from build123d import *

# Parameters (mm, degrees)
SALIENTE_EXTRUIR1_DEPTH  = 38
CORTAR_EXTRUIR1_DEPTH    = 273.053680503
CROQUIS3_R               = 19
SALIENTE_EXTRUIR3_DEPTH  = 26
REDONDEO1_R              = 6
CROQUIS4_R               = 28.5
CORTAR_EXTRUIR2_DEPTH    = 1
REDONDEO1_OF_SIMETR_A1_R = 6
REDONDEO2_R              = 6


with BuildPart() as part:
    # Croquis1 → Saliente-Extruir1 (new, symmetric)
    with BuildSketch(Plane.XY):
        Polygon((0, 0), (0, 139), (38, 139), (127, 50), (127, 0), align=None)
    extrude(amount=SALIENTE_EXTRUIR1_DEPTH, both=True)

    # Croquis2 → Cortar-Extruir1 (cut, through all, along a direction that is not the sketch's normal)
    with BuildSketch(Plane(origin=(0, 139, 0), x_dir=(1, 0, 0), z_dir=(0, 1, 0))):
        Polygon((38, 0), (38, 13), (12, 13), (12, -13), (38, -13), align=None)
    extrude(amount=-CORTAR_EXTRUIR1_DEPTH, dir=(-0.7071067811865515, 0.7071067811865436, 0), mode=Mode.SUBTRACT)

    # Croquis3 → Saliente-Extruir3 (add)
    with BuildSketch(Plane.XZ):
        with BuildLine():
            Line((0, 38), (0, 89))
            ThreePointArc((0, 89), (38, 127), (76, 89))
            Line((76, 89), (76, 38))
            Line((76, 38), (0, 38))
        make_face()
        with Locations((38, 89)):
            Circle(CROQUIS3_R, mode=Mode.SUBTRACT)
    saliente_extruir3 = extrude(amount=-SALIENTE_EXTRUIR3_DEPTH)

    # Redondeo1
    redondeo1_edges = [part.edges().sort_by_distance(p)[0] for p in [
        (38, 26, 127),
        (76, 26, 63.5),
        (0, 26, 63.5),
    ]]
    fillet(redondeo1_edges, radius=REDONDEO1_R)

    # Croquis4 → Cortar-Extruir2 (cut)
    with BuildSketch(Plane(origin=(0, 26, 0), x_dir=(1, 0, 0), z_dir=(0, 1, 0))):
        with Locations(Location((38, -89, 0), (0, 0, 180))):
            Circle(CROQUIS4_R)
    cortar_extruir2 = extrude(amount=-CORTAR_EXTRUIR2_DEPTH, mode=Mode.SUBTRACT)

    # Simetría1: Saliente-Extruir3, Cortar-Extruir2 across plane
    add(saliente_extruir3.mirror(Plane.XY))
    add(cortar_extruir2.mirror(Plane.XY), mode=Mode.SUBTRACT)

    # Redondeo1 of Simetría1
    redondeo1_of_simetr_a1_edges = [part.edges().sort_by_distance(p)[0] for p in [
        (38, 26, -127),
        (76, 26, -63.5),
        (0, 26, -63.5),
    ]]
    fillet(redondeo1_of_simetr_a1_edges, radius=REDONDEO1_OF_SIMETR_A1_R)

    # Redondeo2
    # the kernel refuses this fillet: 6 mm, written as the material it adds along each edge
    with BuildSketch(Plane(origin=(70, 26, 38), x_dir=(0, 0, 1), z_dir=(-1, 0, 0))) as redondeo2_piece_1:
        with BuildLine():
            CenterArc((REDONDEO2_R, REDONDEO2_R), REDONDEO2_R, 180, 90)
            Line((0, REDONDEO2_R), (0, 0))
            Line((0, 0), (REDONDEO2_R, 0))
        make_face()
    extrude(amount=64)
    with BuildSketch(Plane(origin=(76, 0, 38), x_dir=(0, 0, 1), z_dir=(0, 1, 0))) as redondeo2_piece_2:
        with BuildLine():
            CenterArc((REDONDEO2_R, REDONDEO2_R), REDONDEO2_R, 180, 90)
            Line((0, REDONDEO2_R), (0, 0))
            Line((0, 0), (REDONDEO2_R, 0))
        make_face()
    extrude(amount=20)
    with BuildSketch(Plane(origin=(6, 20, 38), x_dir=(0.8017442392976484, -0.5976672776328276, 0), z_dir=(0.5976672776328276, 0.8017442392976484, 0))) as redondeo2_piece_3_section:
        with BuildLine():
            CenterArc((6 + REDONDEO2_R, -REDONDEO2_R), REDONDEO2_R, 90, 90)
            Line((6 + REDONDEO2_R, 0), (6, 0))
            Line((6, 0), (6, -REDONDEO2_R))
        make_face()
    redondeo2_piece_3 = revolve(axis=Axis((6, 20, 38), (0, 0, -1)), revolution_arc=233.296989237, mode=Mode.PRIVATE)
    redondeo2_piece_3 = split(redondeo2_piece_3, bisect_by=Plane(origin=(0, 24.499633638, 39.86976996), z_dir=(1, 0, 0)), keep=Keep.TOP, mode=Mode.PRIVATE)
    add(redondeo2_piece_3)
    with BuildSketch(Plane(origin=(70, 20, 38), x_dir=(1, 0, 0), z_dir=(0, -1, 0))) as redondeo2_piece_4:
        with BuildLine():
            CenterArc((6 + REDONDEO2_R, REDONDEO2_R), REDONDEO2_R, 180, 90)
            Line((6 + REDONDEO2_R, 0), (6, 0))
            Line((6, 0), (6, REDONDEO2_R))
        make_face()
    revolve(axis=Axis((70, 20, 38), (0, 0, 1)), revolution_arc=90)
    with BuildSketch(Plane(origin=(70, 26, -38), x_dir=(0, 0, -1), z_dir=(-1, 0, 0))) as redondeo2_piece_5:
        with BuildLine():
            CenterArc((REDONDEO2_R, -REDONDEO2_R), REDONDEO2_R, 90, 90)
            Line((0, -REDONDEO2_R), (0, 0))
            Line((0, 0), (REDONDEO2_R, 0))
        make_face()
    extrude(amount=64)
    with BuildSketch(Plane(origin=(76, 0, -38), x_dir=(0, 0, -1), z_dir=(0, 1, 0))) as redondeo2_piece_6:
        with BuildLine():
            CenterArc((REDONDEO2_R, -REDONDEO2_R), REDONDEO2_R, 90, 90)
            Line((0, -REDONDEO2_R), (0, 0))
            Line((0, 0), (REDONDEO2_R, 0))
        make_face()
    extrude(amount=20)
    with BuildSketch(Plane(origin=(6, 20, -38), x_dir=(0.8017442392976486, -0.5976672776328271, 0), z_dir=(0.5976672776328271, 0.8017442392976486, 0))) as redondeo2_piece_7_section:
        with BuildLine():
            CenterArc((6 + REDONDEO2_R, REDONDEO2_R), REDONDEO2_R, 180, 90)
            Line((6, REDONDEO2_R), (6, 0))
            Line((6, 0), (6 + REDONDEO2_R, 0))
        make_face()
    redondeo2_piece_7 = revolve(axis=Axis((6, 20, -38), (0, 0, -1)), revolution_arc=233.296989237, mode=Mode.PRIVATE)
    redondeo2_piece_7 = split(redondeo2_piece_7, bisect_by=Plane(origin=(0, 24.499633653, -39.869769899), z_dir=(1, 0, 0)), keep=Keep.TOP, mode=Mode.PRIVATE)
    add(redondeo2_piece_7)
    with BuildSketch(Plane(origin=(70, 20, -38), x_dir=(1, 0, 0), z_dir=(0, -1, 0))) as redondeo2_piece_8:
        with BuildLine():
            CenterArc((6 + REDONDEO2_R, -REDONDEO2_R), REDONDEO2_R, 90, 90)
            Line((6 + REDONDEO2_R, 0), (6, 0))
            Line((6, 0), (6, -REDONDEO2_R))
        make_face()
    revolve(axis=Axis((70, 20, -38), (0, 0, 1)), revolution_arc=90)


solid = part.part
CAD build for the part. Positions are in the model's coordinates, mm. A direction names the side the tool comes from. Round coordinates to 2 decimals unless told otherwise and drop trailing zeros. Loops run counter-clockwise (first coordinate to the right, second up) from the corner with the lowest first, then second, coordinate; pieces in that order, holes last.
(1) Drop flat-ended pins along their axis: pin 1 (6 mm diameter, centred on x = 104.5, y = 18, fed in from +Z); pin 2 (10 mm diameter, centred on x = 49.5, y = 59.5, fed in from -Z); pin 3 (10 mm diameter, centred on y = 6.5, z = -77.5, fed in from +X). Give the stop position or say it passes through.
(2) Which spindle directions (+Z, -Z, +X, -X, +Y, -Y) get a long thin tool onto all of the face, cutting with end or side? Do faces 1 (the flat face through (76, 10, -67)), 2 (the flat face through (19, 25, 83)), 3 (the cylindrical face through (1.804, 24.289, 66.815)). Say none if no direction does.
(3) Cut at A-A (y = 66.5). Give the cut face in (x, z), plus the area to 3 significant figures.
(4) Cut at B-B (z = 5.5). Give the cut face in (x, y), plus the area to 3 significant figures.
(5) Cut at D-D (x = 41). State how many separate pieces and enclosed holes the cut face has, plus the area to 3 significant figures.
(6) Cut at C-C (x = 109). Give the cut face in (y, z).
(7) Wall check: line 1 along Z through (x, y) = (38, 12.25); line 2 along X through (y, z) = (7.75, -89); line 3 along Z through (x, y) = (84, 90). Give the ranges that are in metal, low to high.
(8) Two-plate mould, pull along X, no slides. Class faces 4 (the flat face through (78, 90, 13)), 5 (the cylindrical face through (35.53, 12.32, -107.84)), 6 (the cylindrical face through (37.16, 9.86, 126.99)): +X half, -X half, draft (parallel to the pull), parting line (faces both ways), or undercut.
Findings below:
1. pin 1: stops at z = 38
1. pin 2: stops at z = -38
1. pin 3: stops at x = 76
2. face 1: -Z, +X, +Y, -Y
2. face 2: +Y
2. face 3: +Z, -X, +Y
3. outline: (0, -38) - (110.5, -38) - (110.5, -13) - (84.5, -13) - (84.5, 13) - (110.5, 13) - (110.5, 38) - (0, 38) - close
3. area: 7,720 mm2
4. outline: (0, 0) - (127, 0) - (127, 24) - (12, 139) - (0, 139) - close
4. area: 11,000 mm2
5. separate pieces: 3
5. enclosed holes: 0
5. area: 12,300 mm2
6. outline: (0, -38) - (68, -38) - (68, -13) - (42, -13) - (42, 13) - (68, 13) - (68, 38) - (0, 38) - close
7. line 1: z = -127 to -108, -70 to 70, 108 to 127
7. line 2: x = 0 to 19, 57 to 76
7. line 3: z = -38 to -13, 13 to 38
8. face 4: draft
8. face 5: undercut
8. face 6: parting line
